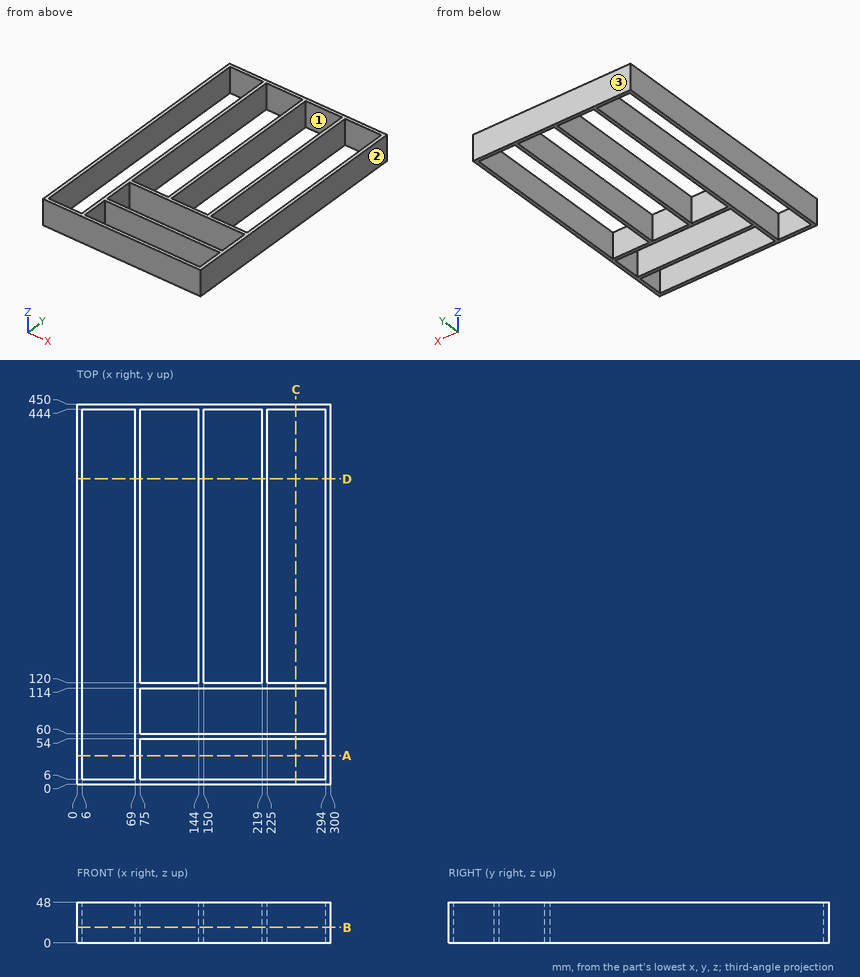
Can you work these out from the drawing? Everything is in mm from the part's minimum corner. Coordinates: 2 decimals unless noted, no trailing zeros. Loops run counter-clockwise (first coordinate to the right, second up) from the corner with the lowest first, then second, coordinate; pieces in that order, holes last. Notation, with made-up numbers: M 73,3.25 L 132,3.25 A27 cw 132,25.25 Z; hole C 29.5,-11.75 d11. An arc over 180 degrees is marked long. One line per item, written item: value.
1. Imagine slicing it at C-C (x = 259). List the corners of the cut face in (y, z) for me.
Geometry says:
outline: M 0,0 L 6,0 L 6,48 L 0,48 Z; M 54,0 L 60,0 L 60,48 L 54,48 Z; M 114,0 L 120,0 L 120,48 L 114,48 Z; M 444,0 L 450,0 L 450,48 L 444,48 Z
2. Imagine slicing it at A-A (y = 34). List the corners of the cut face in (x, z) for me, and give its area (3 significant figures).
Geometry says:
outline: M 0,0 L 6,0 L 6,48 L 0,48 Z; M 69,0 L 75,0 L 75,48 L 69,48 Z; M 294,0 L 300,0 L 300,48 L 294,48 Z
area: 864 mm2
3. Please list where these lines run through material, in increasing order: probe 1 along Y at (x, z) = (151, 4); probe 2 along X at (y, z) = (173.5, 24); probe 3 along Y at (x, z) = (18.5, 6).
Geometry says:
probe 1: y = 0 to 6, 54 to 60, 114 to 120, 444 to 450
probe 2: x = 0 to 6, 69 to 75, 144 to 150, 219 to 225, 294 to 300
probe 3: y = 0 to 6, 444 to 450
4. Thinking about a two-plate mould opening in X: for the marked faces 1, 2 and 3, which applies, +X half, -X half, draft (parallel to the pull), parting line (faces both ways), or undercut?
Geometry says:
face 1: undercut
face 2: +X half
face 3: draft
5. Imagine slicing it at D-D (y = 361.5). List the corners of the cut face in (x, z) for me.
Geometry says:
outline: M 0,0 L 6,0 L 6,48 L 0,48 Z; M 69,0 L 75,0 L 75,48 L 69,48 Z; M 144,0 L 150,0 L 150,48 L 144,48 Z; M 219,0 L 225,0 L 225,48 L 219,48 Z; M 294,0 L 300,0 L 300,48 L 294,48 Z
6. Imagine slicing it at B-B (z = 18.5). List the corners of the cut face in (x, y) for me, and give its area (3 significant figures).
Geometry says:
outline: M 0,0 L 300,0 L 300,450 L 0,450 Z; hole M 6,6 L 69,6 L 69,444 L 6,444 Z; hole M 75,6 L 294,6 L 294,54 L 75,54 Z; hole M 75,60 L 294,60 L 294,114 L 75,114 Z; hole M 75,120 L 144,120 L 144,444 L 75,444 Z; hole M 150,120 L 219,120 L 219,444 L 150,444 Z; hole M 225,120 L 294,120 L 294,444 L 225,444 Z
area: 18,000 mm2
